```python
from build123d import *

# Parameters (mm, degrees)
ESQUISSE1_R        = 1.75
BOSS_EXTRU_1_DEPTH = 180


with BuildPart() as part:
    # Esquisse1 → Boss.-Extru.1 (new body)
    with BuildSketch(Plane.XY):
        with BuildLine():
            Line((-1.5, 5), (-5, 5))
            Line((-5, 5), (-5, 1.5))
            Line((-5, 1.5), (-4, 1.5))
            Line((-4, 1.5), (-4, 2.5))
            Line((-4, 2.5), (-3.207106781, 2.5))
            Line((-3.207106781, 2.5), (-2.216672281, 1.15601211))
            ThreePointArc((-2.216672281, 1.15601211), (-2.5, 0), (-2.216672281, -1.15601211))
            Line((-2.216672281, -1.15601211), (-3.207106781, -2.5))
            Line((-3.207106781, -2.5), (-4, -2.5))
            Line((-4, -2.5), (-4, -1.5))
            Line((-4, -1.5), (-5, -1.5))
            Line((-5, -1.5), (-5, -5))
            Line((-5, -5), (-1.5, -5))
            Line((-1.5, -5), (-1.5, -4))
            Line((-1.5, -4), (-2.5, -4))
            Line((-2.5, -4), (-2.5, -3.207106781))
            Line((-2.5, -3.207106781), (-1.15601211, -2.216672281))
            ThreePointArc((-1.15601211, -2.216672281), (0, -2.5), (1.15601211, -2.216672281))
            Line((1.15601211, -2.216672281), (2.5, -3.207106781))
            Line((2.5, -3.207106781), (2.5, -4))
            Line((2.5, -4), (1.5, -4))
            Line((1.5, -4), (1.5, -5))
            Line((1.5, -5), (5, -5))
            Line((5, -5), (5, -1.5))
            Line((5, -1.5), (4, -1.5))
            Line((4, -1.5), (4, -2.5))
            Line((4, -2.5), (3.207106781, -2.5))
            Line((3.207106781, -2.5), (2.216672281, -1.15601211))
            ThreePointArc((2.216672281, -1.15601211), (2.5, 0), (2.216672281, 1.15601211))
            Line((2.216672281, 1.15601211), (3.207106781, 2.5))
            Line((3.207106781, 2.5), (4, 2.5))
            Line((4, 2.5), (4, 1.5))
            Line((4, 1.5), (5, 1.5))
            Line((5, 1.5), (5, 5))
            Line((5, 5), (1.5, 5))
            Line((1.5, 5), (1.5, 4))
            Line((1.5, 4), (2.5, 4))
            Line((2.5, 4), (2.5, 3.207106781))
            Line((2.5, 3.207106781), (1.15601211, 2.216672281))
            ThreePointArc((1.15601211, 2.216672281), (0, 2.5), (-1.15601211, 2.216672281))
            Line((-1.15601211, 2.216672281), (-2.5, 3.207106781))
            Line((-2.5, 3.207106781), (-2.5, 4))
            Line((-2.5, 4), (-1.5, 4))
            Line((-1.5, 4), (-1.5, 5))
        make_face()
        Polygon((-4.75, 1.75), (-4.75, 4.75), (-1.75, 4.75), (-1.75, 4.25), (-2.75, 4.25), (-2.75, 2.75), (-4.25, 2.75), (-4.25, 1.75), align=None, mode=Mode.SUBTRACT)
        with Locations(Location((0, 0, 0), (0, 0, 180))):
            Circle(ESQUISSE1_R, mode=Mode.SUBTRACT)
        Polygon((-4.75, -4.75), (-4.75, -1.75), (-4.25, -1.75), (-4.25, -2.75), (-2.75, -2.75), (-2.75, -4.25), (-1.75, -4.25), (-1.75, -4.75), align=None, mode=Mode.SUBTRACT)
        Polygon((4.75, 4.75), (4.75, 1.75), (4.25, 1.75), (4.25, 2.75), (2.75, 2.75), (2.75, 4.25), (1.75, 4.25), (1.75, 4.75), align=None, mode=Mode.SUBTRACT)
        Polygon((4.75, -4.75), (1.75, -4.75), (1.75, -4.25), (2.75, -4.25), (2.75, -2.75), (4.25, -2.75), (4.25, -1.75), (4.75, -1.75), align=None, mode=Mode.SUBTRACT)
    extrude(amount=BOSS_EXTRU_1_DEPTH)


solid = part.part
```
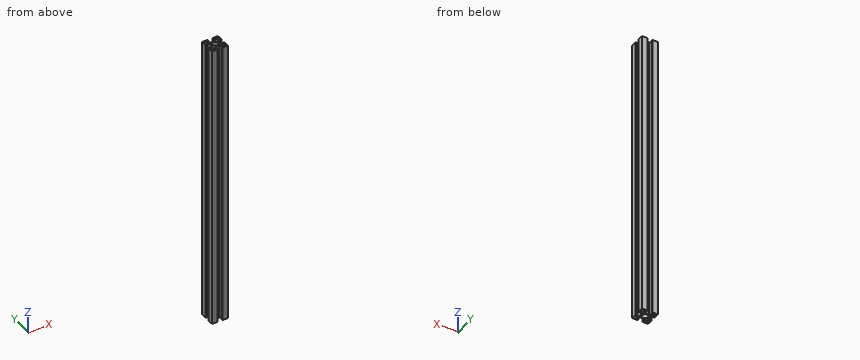
Input: part model. Units: mm. Frame: model coordinates. Coordinates: 2 decimals unless noted, no trailing zeros. Answer in a Markdown table with one row per item.
1. First-contact query: pin 1 (6 mm diameter, centred on y = 0.5, z = 82, fed in from +X). Flat tip, straight axial feed; report the tip coordinate or a pass-through.
Response:
| item | result |
|---|---|
| pin 1 | stops at x = 5 |
2. Material intervals for line 1 (X direction, y = -3.25, z = 128); line 2 (X direction, y = 3, z = 63), sorted ascending.
Response:
| item | result |
|---|---|
| line 1 | x = -5 to -4.75, -2.75 to -2.5, 2.5 to 2.75, 4.75 to 5 |
| line 2 | x = -5 to -4.75, -2.75 to -2.22, 2.22 to 2.75, 4.75 to 5 |
3. Section A-A, the plane z = 135.5. Count the separate pieces of the cut face and the enclosed holes in it, then the cut area to 3 significant figures.
Response:
| item | result |
|---|---|
| separate pieces | 1 |
| enclosed holes | 5 |
| area | 29.8 mm2 |
